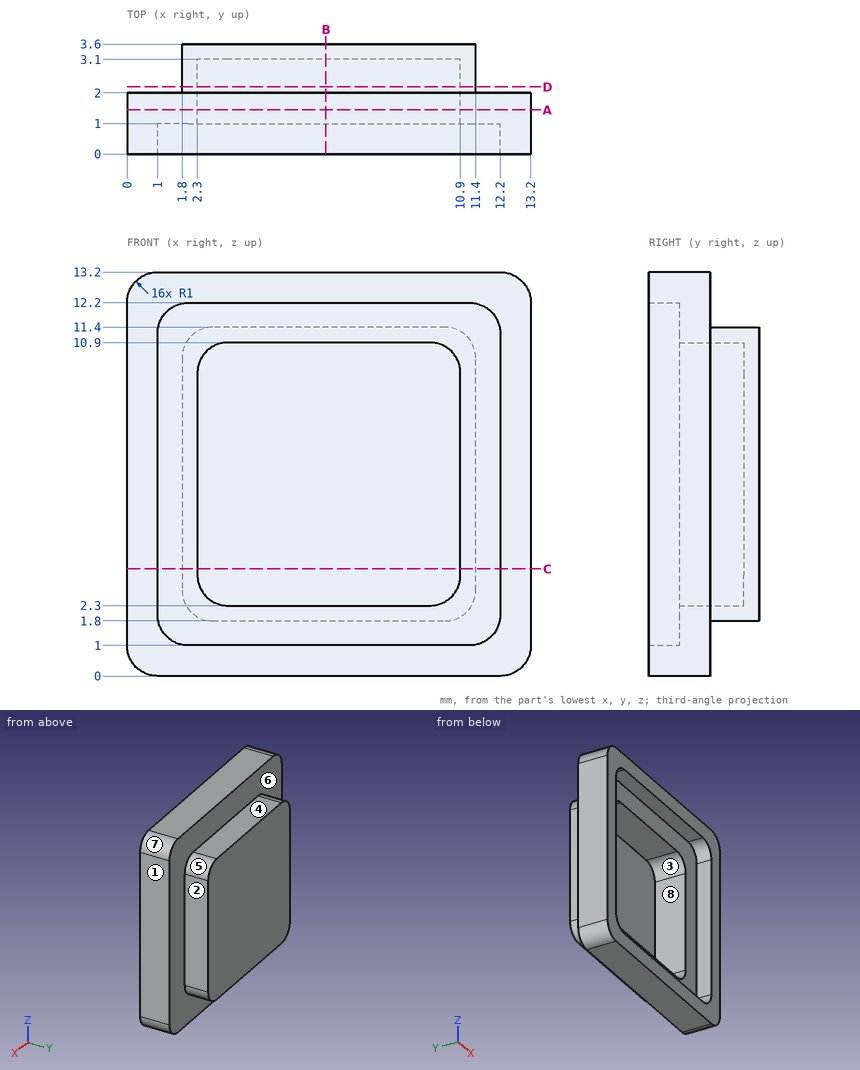
Source: three-view drawing plus pictorial views. Frame: mm from the lowest corner of the part. A direction names the side the tool comes from. Give positions to 0.01 mm unless a question says otherwise; leave off trailing zeros. Order: outer loops, then holes, each group sorted by start corner. A loop starts at its lowest first (then second) coordinate and runs counter-clockwise, first axis right, second up. Notation, with made-up numbers: (-21, 19) - (28, 19) arc R28 ccw to (28, 57) - close; hole circle Ø11 at (60.25, -22). An arc over 180 degrees is marked (long way). Answer as a JSON object with one key per item and string values. Group by question number.
Q1. Set-up query: the marked faces 1, 2, 3, 4 and 5. Return all of +Z, -Z, +X, -X, +Y, -Y with unobstructed straight access to the full face (end or side cutting, diameter ignored); none if empty.
Q2. Cut plane A-A, the plane y = 1.45. Output: boundary loops of the cut face in (x, z), then the cut area to 3 significant figures.
Q3. Cut plane B-B, the plane x = 6.5. Output: boundary loops of the cut face in (y, z), then the cut area to 3 significant figures.
Q4. Line query: probe 1 along Z at (x, y) = (10.75, 0.65); probe 2 along X at (y, z) = (1.55, 6); probe 3 along Z at (x, y) = (6.5, 2.8). Output: solid intervals per line, ascending.
Q5. Cut plane D-D, the plane y = 2.2. Output: boundary loops of the cut face in (x, z), then the cut area to 3 significant figures.
Q6. Mould query, pull axis Z, two halves, no side actions, for the marked faces 6, 7 and 8. Classes: pulls with the +Z half, pulls with the -Z half, needs draft (parallel to the pull), parting line crosses it, or undercut.
Q7. First-contact query: pin 1 Ø1.8 at (y, z) = (3, 8) entering from -X; pin 2 Ø1.8 at (x, y) = (8.5, 3) entering from +Z; pin 3 Ø3 at (x, z) = (8.5, 10) entering from -Y. Flat tips, straight axial feed; report the tip coordinate or a pass-through.
Q8. Cut plane C-C, the plane z = 3.5. Output: boundary loops of the cut face in (x, y), then the cut area to 3 significant figures.
Results:
{
 "1": {"face 1": "+Z, -Z, +X, +Y, -Y", "face 2": "+Z, -Z, +X, +Y", "face 3": "-Y", "face 4": "+Z, +X, -X, +Y", "face 5": "+Z, +X, +Y"},
 "2": {"outline": "(0, 1) arc R1 ccw to (1, 0) - (12.2, 0) arc R1 ccw to (13.2, 1) - (13.2, 12.2) arc R1 ccw to (12.2, 13.2) - (1, 13.2) arc R1 ccw to (0, 12.2) - close; hole (2.3, 3.3) arc R1 ccw to (3.3, 2.3) - (9.9, 2.3) arc R1 ccw to (10.9, 3.3) - (10.9, 9.9) arc R1 ccw to (9.9, 10.9) - (3.3, 10.9) arc R1 ccw to (2.3, 9.9) - close", "area": "100 mm^2"},
 "3": {"outline": "(0, 0) - (2, 0) - (2, 1.8) - (3.6, 1.8) - (3.6, 11.4) - (2, 11.4) - (2, 13.2) - (0, 13.2) - (0, 12.2) - (1, 12.2) - (1, 10.9) - (3.1, 10.9) - (3.1, 2.3) - (1, 2.3) - (1, 1) - (0, 1) - close", "area": "12.5 mm^2"},
 "4": {"probe 1": "0 to 1, 12.2 to 13.2", "probe 2": "0 to 2.3, 10.9 to 13.2", "probe 3": "1.8 to 2.3, 10.9 to 11.4"},
 "5": {"outline": "(1.8, 2.8) arc R1 ccw to (2.8, 1.8) - (10.4, 1.8) arc R1 ccw to (11.4, 2.8) - (11.4, 10.4) arc R1 ccw to (10.4, 11.4) - (2.8, 11.4) arc R1 ccw to (1.8, 10.4) - close; hole (2.3, 3.3) arc R1 ccw to (3.3, 2.3) - (9.9, 2.3) arc R1 ccw to (10.9, 3.3) - (10.9, 9.9) arc R1 ccw to (9.9, 10.9) - (3.3, 10.9) arc R1 ccw to (2.3, 9.9) - close", "area": "18.2 mm^2"},
 "6": {"face 6": "needs draft", "face 7": "pulls with the +Z half", "face 8": "undercut"},
 "7": {"pin 1": "x = 1.8", "pin 2": "z = 11.4", "pin 3": "y = 1"},
 "8": {"outline": "(0, 0) - (1, 0) - (1, 1) - (2.3, 1) - (2.3, 3.1) - (10.9, 3.1) - (10.9, 1) - (12.2, 1) - (12.2, 0) - (13.2, 0) - (13.2, 2) - (11.4, 2) - (11.4, 3.6) - (1.8, 3.6) - (1.8, 2) - (0, 2) - close", "area": "12.5 mm^2"}
}
